from build123d import *

# Parameters (mm, degrees)
SKETCH1_R               = 5
BOSS_EXTRUDE1_DEPTH     = 119.147
CUT_EXTRUDE1_REACH      = 121.357
SKETCH2_R               = 4
CUT_EXTRUDE2_DEPTH      = 120.356640406
CUT_EXTRUDE2_DEPTH_BACK = 120.356640406
SKETCH5_R               = 1.5


with BuildPart() as part:
    # Sketch1 → Boss-Extrude1 (new body)
    with BuildSketch(Plane.XY):
        Circle(SKETCH1_R)
    extrude(amount=BOSS_EXTRUDE1_DEPTH)

    # Sketch2 → Cut-Extrude1 (cut, up to next)
    with BuildSketch(Plane.XY.offset(119.147), mode=Mode.PRIVATE) as cut_extrude1_sk1:
        Circle(SKETCH2_R)
    cut_extrude1_tool1 = extrude(cut_extrude1_sk1.sketch, amount=-CUT_EXTRUDE1_REACH, mode=Mode.PRIVATE) & part.part
    add(cut_extrude1_tool1.solids().sort_by_distance((0, 0, 119.147))[0], mode=Mode.SUBTRACT)

    # Sketch5 → Cut-Extrude2 (cut, two sides: drawn at the far end of the back side and taken through both)
    with BuildSketch(Plane(origin=(0, 0, 0), x_dir=(1, 0, 0), z_dir=(0, 1, 0)).offset(-CUT_EXTRUDE2_DEPTH_BACK)):
        with Locations(Location((0, -26.689, 0), (0, 0, 270))):
            Circle(SKETCH5_R)
        with Locations(Location((0, -92.458, 0), (0, 0, 270))):
            Circle(SKETCH5_R)
    extrude(amount=CUT_EXTRUDE2_DEPTH + CUT_EXTRUDE2_DEPTH_BACK, mode=Mode.SUBTRACT)


solid = part.part
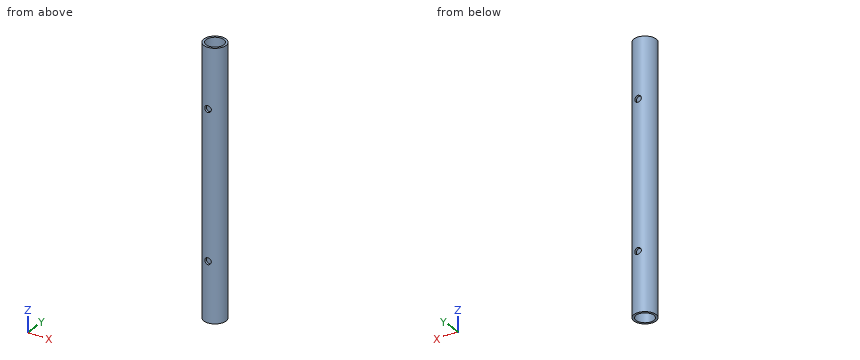
Input: part model. Units: mm. Frame: model coordinates. Give positions to 0.01 mm unless a question says otherwise; leave off trailing zeros. Loops run counter-clockwise (first coordinate to the right, second up) from the corner with the lowest first, then second, coordinate; pieces in that order, holes last. Notation, with made-up numbers: M 87.5,40.25 L 95.5,40.25 A23 cw 95.5,71.25 Z; hole C 30,-0.75 d1. An arc over 180 degrees is marked long. Use CSV: the item, a comma, the result in double quotes.
(1) Section C-C, the plane z = 57. Return loops of the section in (x, y).
Outcome:
outline,"C 0,0 d10; hole C 0,0 d8"
(2) Section B-B, the plane x = 0. Return loops of the section in (y, z), plus the area to 3 significant figures.
Outcome:
outline,"M -5,0 L -4,0 L -4,25.19 L -5,25.19 Z; M -5,28.19 L -4,28.19 L -4,90.96 L -5,90.96 Z; M -5,93.96 L -4,93.96 L -4,119.15 L -5,119.15 Z; M 4,0 L 5,0 L 5,25.19 L 4,25.19 Z; M 4,28.19 L 5,28.19 L 5,90.96 L 4,90.96 Z; M 4,93.96 L 5,93.96 L 5,119.15 L 4,119.15 Z"
area,"226 mm²"
(3) Pin query (flat end, axial travel): P1, Ø2, axis at y = -4, z = 68.5, coming from the +X side; P2, Ø1.5, axis at x = 1.5, z = 34, coming from the -Y side; P3, Ø1.5, axis at y = -1.5, z = 60, coming from the -X side. Return the tip coordinate at first contact, or that it passes through.
Outcome:
P1,"stops at x = 4"
P2,"stops at y = -4.94"
P3,"stops at x = -4.94"
(4) Material intervals for L1, parallel to Z at x = 0, y = -4.55; L2, parallel to Z at x = -1, y = -4; L3, parallel to Y at x = 0, z = 28.5, sorted ascending. Write a range as [from, to].
Outcome:
L1,"z = [0, 25.19], [28.19, 90.96], [93.96, 119.15]"
L2,"z = [0, 25.57], [27.81, 91.34], [93.58, 119.15]"
L3,"y = [-5, -4], [4, 5]"
(5) Section A-A, the plane y = 0. Return loops of the section in (x, z), plus the area to 3 significant figures.
Outcome:
outline,"M -5,0 L -4,0 L -4,119.15 L -5,119.15 Z; M 4,0 L 5,0 L 5,119.15 L 4,119.15 Z"
area,"238 mm²"
